```python
from build123d import *

# Parameters (mm, degrees)
SKETCH2_W           = 44
SKETCH2_H           = 4
SKETCH2_W_2         = 4
SKETCH2_W_3         = 26.15
SKETCH2_W_4         = 25.56
BOSS_EXTRUDE1_DEPTH = 70
FILLET1_R           = 1.5
SKETCH3_R           = 3
CUT_EXTRUDE1_DEPTH  = 95.313214875
SKETCH4_R           = 5
CUT_EXTRUDE2_DEPTH  = 1.4


with BuildPart() as part:
    # Sketch2 → Boss-Extrude1 (new body)
    with BuildSketch(Plane(origin=(0, 0, 0), x_dir=(0, 0, -1), z_dir=(1, 0, 0))):
        with Locations((-2, 0)):
            Rectangle(SKETCH2_W, SKETCH2_H)
        with Locations((22, 0)):
            Rectangle(SKETCH2_W_2, SKETCH2_H)
        Polygon((24, -2), (20, -2), (20, -24.01), (24, -24.01), (24, -20.01), align=None)
        with Locations((37.075, -22.01)):
            Rectangle(SKETCH2_W_3, SKETCH2_H)
        Polygon((50.15, 30.6), (50.15, -20.01), (50.15, -24.01), (54.15, -24.01), (54.15, 34.6), (50.15, 34.6), align=None)
        with Locations((37.37, 32.6)):
            Rectangle(SKETCH2_W_4, SKETCH2_H)
    extrude(amount=BOSS_EXTRUDE1_DEPTH)

    # Fillet1
    fillet1_edges = [part.edges().sort_by_distance(p)[0] for p in [
        (35, -20.01, -24),
        (35, -20.01, -50.15),
        (35, 30.6, -50.15),
    ]]
    fillet(fillet1_edges, radius=FILLET1_R)

    # Sketch3 → Cut-Extrude1 (cut, through all)
    with BuildSketch(Plane(origin=(0, 2, 0), x_dir=(1, 0, 0), z_dir=(0, 1, 0))):
        with Locations(Location((35, 0, 0), (0, 0, 270))):
            Circle(SKETCH3_R)
    extrude(amount=-CUT_EXTRUDE1_DEPTH, mode=Mode.SUBTRACT)

    # Sketch4 → Cut-Extrude2 (cut)
    with BuildSketch(Plane(origin=(0, -2, 0), x_dir=(1, 0, 0), z_dir=(0, 1, 0))):
        with Locations(Location((35, 0, 0), (0, 0, 270))):
            Circle(SKETCH4_R)
    extrude(amount=CUT_EXTRUDE2_DEPTH, mode=Mode.SUBTRACT)


solid = part.part
```
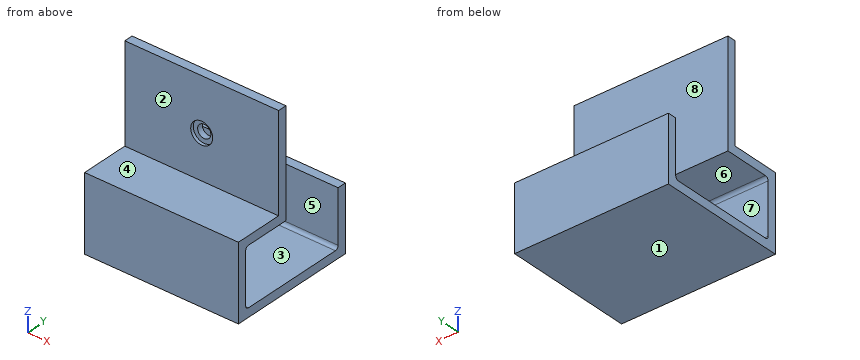
Here's how the part is built. I have some questions about the finished solid (model axes, mm). Face numbers are marked on the shaded views. A direction names the side the tool comes from. Coordinates: 2 decimals unless noted, no trailing zeros. Write each loop counter-clockwise with the first axis right and the second up, starting at its lowest first coordinate (ties: lowest second). Pieces come first, ordered by that corner, then holes. Notation, with made-up numbers: (74.25, 56.25) -> (78.25, 56.25) arc R29 ccw to (78.25, 86.25) -> close; hole circle Ø6 at (22.25, 65.25). An arc over 180 degrees is marked (long way). Use a Markdown table: item, result. Add a question column.
(1) We'd pull the mould along Y, two halves only. Please class the marked faces 1, 2 and 3: +Y half, -Y half, draft (parallel to the pull), parting line (faces both ways), or undercut.
(2) Please list where these lines run through material, in increasing order: line 1 (X direction, y = 0, z = 0); line 2 (Z direction, x = 55.5, y = -10); line 3 (Y direction, x = 41, z = -33.5).
(3) I'm going to push flat-ended pins straight in: P1, Ø2, axis at x = 20.5, z = 2.5, coming from the +Y side; P2, Ø24, axis at x = 37.5, y = 15.5, coming from the +Z side; P3, Ø1.2, axis at x = 25, y = 33.5, coming from the +Z side. Where does each tip first touch, or does it pass through?
(4) If we section it at B-B, the plane x = 35: Write out the boundary of the cut face in (y, z), and give its area (3 significant figures).
(5) If we section it at A-A, the plane z = -32: Write out the boundary of the cut face in (x, y), and give its area (3 significant figures).
(6) If we section it at D-D, the plane x = 9: Write out the boundary of the cut face in (y, z), and give its area (3 significant figures).
(7) For the marked faces 4, 5, 6, 7 and 8, which set-ups out of +Z, -Z, +X, -X, +Y, -Y let a thin tool reach every point of the face, with its end or its side?
(8) If we section it at C-C, the plane y = -3.5: Write out the boundary of the cut face in (x, z), and give its area (3 significant figures).
Outcome:
| question | item | result |
|---|---|---|
| 1 | face 1 | draft |
| 1 | face 2 | -Y half |
| 1 | face 3 | undercut |
| 2 | line 1 | x = 0 to 32, 38 to 70 |
| 2 | line 2 | z = -54.15 to -50.15, -24 to -20 |
| 2 | line 3 | y = -24.01 to -20.01, 30.6 to 34.6 |
| 3 | P1 | stops at y = 2 |
| 3 | P2 | stops at z = -50.15 |
| 3 | P3 | stops at z = -24.59 |
| 4 | outline | (-24.01, -54.15) -> (34.6, -54.15) -> (34.6, -24.59) -> (30.6, -24.59) -> (30.6, -48.65) arc R1.5 cw to (29.1, -50.15) -> (-18.51, -50.15) arc R1.5 cw to (-20.01, -48.65) -> (-20.01, -25.5) arc R1.5 cw to (-18.51, -24) -> (2, -24) -> (2, -3) -> (-0.6, -3) -> (-0.6, -5) -> (-2, -5) -> (-2, -20) -> (-24.01, -20) -> close; (-2, 5) -> (-0.6, 5) -> (-0.6, 3) -> (2, 3) -> (2, 24) -> (-2, 24) -> close |
| 4 | area | 693 mm^2 |
| 5 | outline | (0, -24.01) -> (70, -24.01) -> (70, -20.01) -> (0, -20.01) -> close; (0, 30.6) -> (70, 30.6) -> (70, 34.6) -> (0, 34.6) -> close |
| 5 | area | 560 mm^2 |
| 6 | outline | (-24.01, -54.15) -> (34.6, -54.15) -> (34.6, -24.59) -> (30.6, -24.59) -> (30.6, -48.65) arc R1.5 cw to (29.1, -50.15) -> (-18.51, -50.15) arc R1.5 cw to (-20.01, -48.65) -> (-20.01, -25.5) arc R1.5 cw to (-18.51, -24) -> (2, -24) -> (2, 24) -> (-2, 24) -> (-2, -20) -> (-24.01, -20) -> close |
| 6 | area | 723 mm^2 |
| 7 | face 4 | +Z, +X, -X, -Y |
| 7 | face 5 | +Z, +X, -X |
| 7 | face 6 | +X, -X, +Y |
| 7 | face 7 | +X, -X |
| 7 | face 8 | +Z, +X, -X, +Y |
| 8 | outline | (0, -54.15) -> (70, -54.15) -> (70, -50.15) -> (0, -50.15) -> close; (0, -24) -> (70, -24) -> (70, -20) -> (0, -20) -> close |
| 8 | area | 560 mm^2 |
